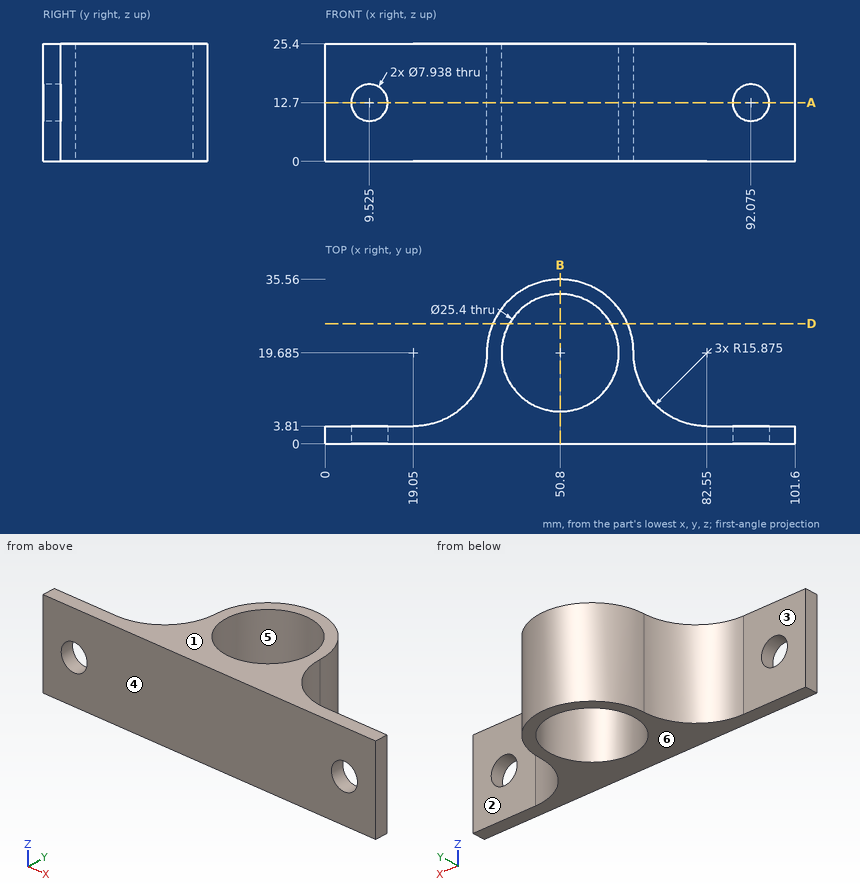
Print and shaded views of the part. All mm, measured from the part's lowest x, y and z. A direction names the side the tool comes from. Coordinates: 2 decimals unless noted, no trailing zeros. Write each loop counter-clockwise with the first axis right and the second up, starting at its lowest first coordinate (ties: lowest second). Pieces come first, ordered by that corner, then holes. Notation, with made-up numbers: (45, 6) -> (104, 6) arc R15 ccw to (104, 17) -> close; hole circle Ø8 at (17, 15). An arc over 180 degrees is marked (long way). Use CSV: the item, a comma, the result in double quotes. Start each with the question number.
Q1. Cut at A-A, the plane z = 12.7. State how many separate pieces and enclosed holes the cut face has, then the cut area to 3 significant figures.
Q2. 3-axis set-ups, long thin cutter, end or side, ignore diameter. For the marked faces 1, 2 and 3: which of +Z, -Z, +X, -X, +Y, -Y reach the whole face in a straight line?
Q3. Drill centre lines: probe 1 along X at (y, z) = (19, 13.5); probe 2 along Y at (x, z) = (50.8, 10.25) (1 decimal); probe 3 along Y at (x, z) = (55, 4.5) (1 decimal). Where is each one in solid material? Low to high.
Q4. Flat gauge pins, fed straight in: pin 1 Ø15 at (x, z) = (12, 16.5) entering from +Y; pin 2 Ø1 at (x, z) = (52, 20) entering from +Y (1 decimal); pin 3 Ø4 at (y, z) = (18.5, 6.5) entering from -X. Where does each tip first touch, or does it go through?
Q5. Pull direction Y, two halves, no side cores. Call the marked faces 4, 5 and 6: released by +Y, released by -Y, zero draft, split by the parting line, or undercut.
Q6. Cut at B-B, the plane x = 50.8. List the corners of the cut face in (y, z) (1 decimal), then the cut area to 3 significant figures.
Q7. Cut at D-D, the plane y = 26. List the corners of the cut face in (x, z) (1 decimal), then the cut area to 3 significant figures.
Checked values:
1,separate pieces,"3"
1,enclosed holes,"1"
1,area,"828 mm²"
2,face 1,"+Z, +X, -X, +Y, -Y"
2,face 2,"+Z, -Z, +X, +Y"
2,face 3,"+Z, -Z, -X, +Y"
3,probe 1,"x = 34.91 to 38.12, 63.48 to 66.69"
3,probe 2,"y = 0 to 7, 32.4 to 35.6"
3,probe 3,"y = 0 to 7.7, 31.7 to 35"
4,pin 1,"stops at y = 3.82"
4,pin 2,"stops at y = 35.5"
4,pin 3,"stops at x = 34.6"
5,face 4,"released by -Y"
5,face 5,"undercut"
5,face 6,"zero draft"
6,outline,"(0, 0) -> (7, 0) -> (7, 25.4) -> (0, 25.4) -> close; (32.4, 0) -> (35.6, 0) -> (35.6, 25.4) -> (32.4, 25.4) -> close"
6,area,"258 mm²"
7,outline,"(36.2, 0) -> (39.8, 0) -> (39.8, 25.4) -> (36.2, 25.4) -> close; (61.8, 0) -> (65.4, 0) -> (65.4, 25.4) -> (61.8, 25.4) -> close"
7,area,"180 mm²"
